For this review, take the finished solid that the model builds, in its own axes (mm). A direction names the side the tool comes from. Coordinates: 2 decimals unless noted, no trailing zeros. Write each loop counter-clockwise with the first axis right and the second up, starting at its lowest first coordinate (ties: lowest second). Pieces come first, ordered by that corner, then holes. Notation, with made-up numbers: (8.25, 25.5) - (51.25, 25.5) arc R25 cw to (51.25, 59.5) - close; hole circle Ø2 at (85, -32.75). An arc over 180 degrees is marked (long way). Use one line per item in the form item = value. Start each with the question number.
1) We need section C-C (z = 21.75). Give the boundary of the cut face in (x, y), plus the area to 3 significant figures.
2) Tool access review of faces 1 (the flat face through (1, 58, 12)), 2 (the flat face through (1, 6, 23)): name each direction out of +Z, -Z, +X, -X, +Y, -Y from which nothing blocks a thin tool from reaching the whole face with its end or side.
3) Mouldability with a two-part tool opening along X and no side actions: class faces 3 (the cylindrical face through (1, 29, -2)), 4 (the cylindrical face through (0.7, 28.6, -1.4)), 5 (the flat face through (0, 29, 11)) as pulls with the +X half, pulls with the -X half, needs draft (parallel to the pull), parting line crosses it, or undercut.
4) Insertion check: P1, Ø1, axis at x = 0.5, y = 47, coming from the -Z side. The pin has a flat end and moves straight along its axis. Give the tip position at first contact, or say it passes through.
5) We need section A-A (x = 1). Give the boundary of the cut face in (y, z).
6) We need section D-D (z = 13). Give the boundary of the cut face in (x, y), plus the area to 3 significant figures.
7) We need section B-B (y = 42). Give the boundary of the cut face in (x, z).
8) For L1, parallel to X at y = 28.5, z = -1; L2, parallel to Y at x = 0.35, z = 21; L3, parallel to Z at x = 0.8, y = 3, list the stretches that pass through material, from the lowest coordinate up. Write a range as from..to.
```python
from build123d import *

# Parameters (mm, degrees)
EXTRUDE_1_DEPTH = 2
SKETCH_2_R      = 0.5
EXTRUDE_2_DEPTH = 58
SKETCH_3_R      = 0.5
EXTRUDE_3_DEPTH = 52


with BuildPart() as part:
    # Эскиз1 → Бобышка-Вытянуть1 (new body)
    with BuildSketch(Plane(origin=(0, 0, 0), x_dir=(0, 0, -1), z_dir=(1, 0, 0))):
        Polygon((-23, 6), (-20.034972426, 6), (-11.466084386, 0), (0, 0), (0, 58), (-23, 58), align=None)
    extrude(amount=EXTRUDE_1_DEPTH)

    # Эскиз2 → Бобышка-Вытянуть2 (add)
    with BuildSketch(Plane(origin=(0, 0, 0), x_dir=(1, 0, 0), z_dir=(0, 1, 0))):
        with BuildLine():
            Line((0, 1), (0, 0))
            Line((0, 0), (2, 0))
            Line((2, 0), (2, 1))
            ThreePointArc((2, 1), (1, 2), (0, 1))
        make_face()
        with Locations(Location((1, 1, 0), (0, 0, 270))):
            Circle(SKETCH_2_R, mode=Mode.SUBTRACT)
    extrude(amount=EXTRUDE_2_DEPTH)

    # Эскиз3 → Бобышка-Вытянуть3 (add)
    with BuildSketch(Plane.XZ.offset(-6)):
        with BuildLine():
            Line((0, 23), (0, 24))
            ThreePointArc((0, 24), (1, 25), (2, 24))
            Line((2, 24), (2, 23))
            Line((2, 23), (0, 23))
        make_face()
        with Locations(Location((1, 24, 0), (0, 0, 270))):
            Circle(SKETCH_3_R, mode=Mode.SUBTRACT)
    extrude(amount=-EXTRUDE_3_DEPTH)


solid = part.part
```
Determined:
q1.outline = (0, 6) - (2, 6) - (2, 58) - (0, 58) - close
q1.area = 104 mm²
q2.face_1 = +Z, -Z, +X, -X, +Y
q2.face_2 = +Z, +X, -X, -Y
q3.face_3 = parting line crosses it
q3.face_4 = undercut
q3.face_5 = pulls with the -X half
q4.P1 = -2
q5.outline = (0, -2) - (58, -2) - (58, -1.5) - (0, -1.5) - close; (0, -0.5) - (58, -0.5) - (58, 23.5) - (6, 23.5) - (6, 20.03) - (0, 11.47) - close; (6, 24.5) - (58, 24.5) - (58, 25) - (6, 25) - close
q6.outline = (0, 1.07) - (2, 1.07) - (2, 58) - (0, 58) - close
q6.area = 114 mm²
q7.outline = (0, -1) arc R1 ccw to (2, -1) - (2, 24) arc R1 ccw to (0, 24) - close; hole circle Ø1 at (1, -1); hole circle Ø1 at (1, 24)
q8.L1 = 0..0.5, 1.5..2
q8.L2 = 6..58
q8.L3 = -1.98..-1.46, -0.54..15.75
